For this review, take the finished solid that the model builds, in its own axes (mm). Face numbers are marked on the shaded views. A direction names the side the tool comes from. Round coordinates to 2 decimals unless told otherwise and drop trailing zeros. Loops run counter-clockwise (first coordinate to the right, second up) from the corner with the lowest first, then second, coordinate; pieces in that order, holes last.
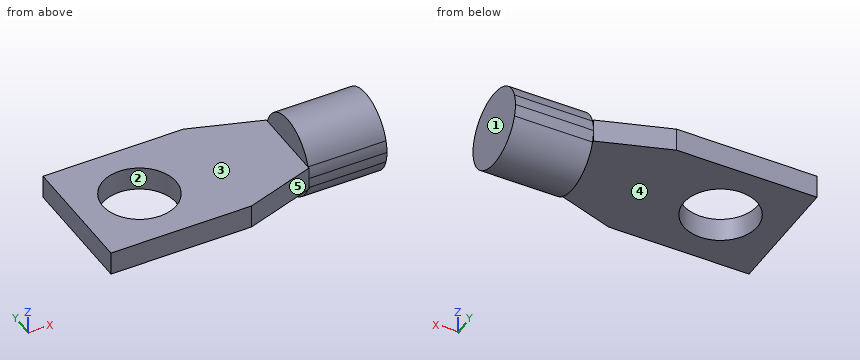
```python
from build123d import *

# Parameters (mm, degrees)
F0_R     = 23.5
F1_DEPTH = 15
F3_DEPTH = 50


with BuildPart() as f1:
    # F0 (on Top) → F1 (new body)
    with BuildSketch(Plane.XY):
        Polygon((-90, -40), (0, -40), (45, -25), (45, 25), (0, 40), (-90, 40), align=None)
        with Locations((-50, 0)):
            Circle(F0_R, mode=Mode.SUBTRACT)
    extrude(amount=F1_DEPTH)

    # F2 (on face) → F3 (join)
    with BuildSketch(Plane.YZ.offset(45)):
        with BuildLine():
            ThreePointArc((23.8484800354, 0), (24.7104431454, 3.7060575179), (25, 7.5))
            ThreePointArc((25, 7.5), (24.7104431454, 11.2939424821), (23.8484800354, 15))
            Line((23.8484800354, 15), (-23.8484800354, 15))
            ThreePointArc((-23.8484800354, 15), (-24.7104431454, 11.2939424821), (-25, 7.5))
            ThreePointArc((-25, 7.5), (-24.7104431454, 3.7060575179), (-23.8484800354, 0))
            Line((-23.8484800354, 0), (23.8484800354, 0))
        make_face()
        with BuildLine():
            Line((-23.8484800354, 15), (23.8484800354, 15))
            ThreePointArc((23.8484800354, 15), (0, 32.5), (-23.8484800354, 15))
        make_face()
        with BuildLine():
            ThreePointArc((-23.8484800354, 0), (0, -17.5), (23.8484800354, 0))
            Line((23.8484800354, 0), (-23.8484800354, 0))
        make_face()
    extrude(amount=F3_DEPTH)


solid = f1.part
```
(1) Add section D-D (y = 14.5). Give the boundary of the cut face in (x, z).
(2) Add section A-A (y = 0). Give the boundary of the cut face in (x, z), plus the area to 3 significant figures.
(3) Add section B-B (x = -50). Give the boundary of the cut face in (y, z), plus the area to 3 significant figures.
(4) For L1, parallel to Y at x = -50, z = 5.5; L2, parallel to Y at x = -44.5, z = 0.5; L3, parallel to Z at x = 4, y = -11, list the stretches that pass through material, from the lowest coordinate up.
(5) The part is to be moulded in two halves that separate along X. For the marked faces 1, 2 and 3, say which applies: pulls with the +X half, pulls with the -X half, needs draft (parallel to the pull), parting line crosses it, or undercut.
(6) For the marked faces 4 and 5, list the 3-axis set-ups (+Z, -Z, +X, -X, +Y, -Y) from which the entire face can be reached by the end or side of a thin tool; tool diameter is ignored.
(7) Insertion check: pin 1 Ø5 at (x, z) = (45, -7.5) entering from +Y; pin 2 Ø19 at (y, z) = (6, 22.5) entering from -X; pin 3 Ø4 at (x, y) = (-62.5, -17) entering from -Z; pin 4 Ø5 at (y, z) = (8.5, -7.5) entering from -X. Each pin has a flat end and moves straight along its axis. Give the tip position at first contact, or say it passes through.
(8) Add section C-C (z = 13). Give the boundary of the cut face in (x, y), plus the area to 3 significant figures.
Outcome:
1. outline: (-90, 0) - (-68.49, 0) - (-68.49, 15) - (-90, 15) - close; (-31.51, 0) - (45, 0) - (45, -12.87) - (95, -12.87) - (95, 27.87) - (45, 27.87) - (45, 15) - (-31.51, 15) - close
2. outline: (-90, 0) - (-73.5, 0) - (-73.5, 15) - (-90, 15) - close; (-26.5, 0) - (45, 0) - (45, -17.5) - (95, -17.5) - (95, 32.5) - (45, 32.5) - (45, 15) - (-26.5, 15) - close
2. area: 3,820 mm2
3. outline: (-40, 0) - (-23.5, 0) - (-23.5, 15) - (-40, 15) - close; (23.5, 0) - (40, 0) - (40, 15) - (23.5, 15) - close
3. area: 495 mm2
4. L1: y = -40 to -23.5, 23.5 to 40
4. L2: y = -40 to -22.85, 22.85 to 40
4. L3: z = 0 to 15
5. face 1: pulls with the +X half
5. face 2: undercut
5. face 3: needs draft
6. face 4: -Z, -X, +Y, -Y
6. face 5: +Z, -Z, +X, -Y
7. pin 1: stops at y = 21.65
7. pin 2: stops at x = -90
7. pin 3: passes through
7. pin 4: stops at x = 45
8. outline: (-90, -40) - (0, -40) - (45, -25) - (45, -24.39) - (95, -24.39) - (95, 24.39) - (45, 24.39) - (45, 25) - (0, 40) - (-90, 40) - close; hole circle Ø47 at (-50, 0)
8. area: 10,800 mm2
